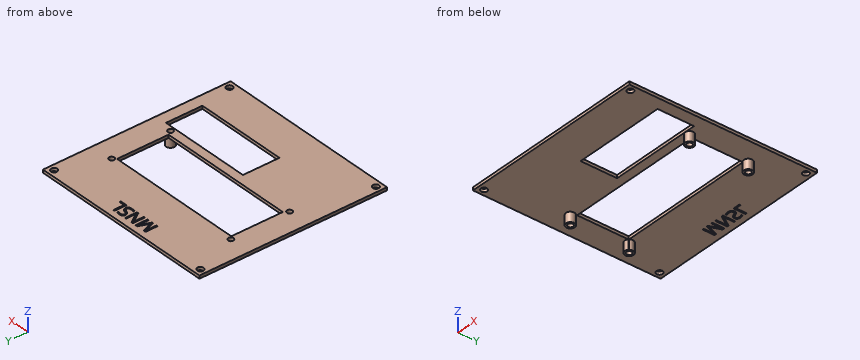
```python
from build123d import *

# Parameters (mm, degrees)
F0_W     = 98.044
F0_H     = 98.044
F0_R     = 1.651
F0_R_2   = 2.286
F0_R_3   = 1.397
F1_DEPTH = 1.5875
F2_DEPTH = 5.08


with BuildPart() as f1:
    # F0 (on Top) → F1 (new body)
    with BuildSketch(Plane.XY):
        Rectangle(F0_W, F0_H)
        with Locations((-45.847, -45.847)):
            Circle(F0_R, mode=Mode.SUBTRACT)
        with Locations((-37.338, -7.874)):
            Circle(F0_R_2, mode=Mode.SUBTRACT)
        with Locations((45.847, -45.847)):
            Circle(F0_R, mode=Mode.SUBTRACT)
        Polygon((-5.334, -29.21), (-5.334, -10.16), (37.3379999666, -10.16), (42.926, -10.16), (42.926, -29.21), align=None, mode=Mode.SUBTRACT)
        with BuildLine():
            ThreePointArc((39.624, -7.874), (38.95444609, -9.4904461136), (37.3379999666, -10.16))
            ThreePointArc((37.3379999666, -10.16), (35.72155391, -6.2575538864), (39.624, -7.874))
        make_face(mode=Mode.SUBTRACT)
        with Locations((-45.847, 45.847)):
            Circle(F0_R, mode=Mode.SUBTRACT)
        with BuildLine():
            Line((-7.9581705729, 39.497), (-8.5479709201, 39.497))
            Line((-8.5479709201, 39.497), (-10.6839301215, 45.0780546875))
            Line((-10.6839301215, 45.0780546875), (-10.7183810764, 45.0780546875))
            add(Edge.make_bspline(
                [(-10.7183810764, 45.0780546875), (-10.6577473958, 44.415218316), (-10.6577473958, 43.5015789931)],
                knots=[0, 0, 0, 1, 1, 1], degree=2))
            Line((-10.6577473958, 43.5015789931), (-10.6577473958, 39.497))
            Line((-10.6577473958, 39.497), (-11.3343641493, 39.497))
            Line((-11.3343641493, 39.497), (-11.3343641493, 45.7932565104))
            Line((-11.3343641493, 45.7932565104), (-10.2319335938, 45.7932565104))
            Line((-10.2319335938, 45.7932565104), (-8.2379123264, 40.5994305556))
            Line((-8.2379123264, 40.5994305556), (-8.2034613715, 40.5994305556))
            Line((-8.2034613715, 40.5994305556), (-6.1929036458, 45.7932565104))
            Line((-6.1929036458, 45.7932565104), (-5.0987413194, 45.7932565104))
            Line((-5.0987413194, 45.7932565104), (-5.0987413194, 39.497))
            Line((-5.0987413194, 39.497), (-5.8304796007, 39.497))
            Line((-5.8304796007, 39.497), (-5.8304796007, 43.5539444444))
            add(Edge.make_bspline(
                [(-5.8304796007, 43.5539444444), (-5.8304796007, 44.2512317708), (-5.7698459201, 45.0697864583)],
                knots=[0, 0, 0, 1, 1, 1], degree=2))
            Line((-5.7698459201, 45.0697864583), (-5.804296875, 45.0697864583))
            Line((-5.804296875, 45.0697864583), (-7.9581705729, 39.497))
        make_face(mode=Mode.SUBTRACT)
        with BuildLine():
            Line((1.5461588542, 45.7932565104), (1.5461588542, 39.497))
            Line((1.5461588542, 39.497), (0.7110677083, 39.497))
            Line((0.7110677083, 39.497), (-2.7298936632, 44.7803984375))
            Line((-2.7298936632, 44.7803984375), (-2.7643446181, 44.7803984375))
            add(Edge.make_bspline(
                [(-2.7643446181, 44.7803984375), (-2.6954427083, 43.8502226563), (-2.6954427083, 43.075765191)],
                knots=[0, 0, 0, 1, 1, 1], degree=2))
            Line((-2.6954427083, 43.075765191), (-2.6954427083, 39.497))
            Line((-2.6954427083, 39.497), (-3.3720594618, 39.497))
            Line((-3.3720594618, 39.497), (-3.3720594618, 45.7932565104))
            Line((-3.3720594618, 45.7932565104), (-2.5452365451, 45.7932565104))
            Line((-2.5452365451, 45.7932565104), (0.8874565972, 40.5305286458))
            Line((0.8874565972, 40.5305286458), (0.9219075521, 40.5305286458))
            add(Edge.make_bspline(
                [(0.9219075521, 40.5305286458), (0.9136393229, 40.6462838542), (0.8833224826, 41.2774253472)],
                knots=[0, 0, 0, 1, 1, 1], degree=2))
            add(Edge.make_bspline(
                [(0.8833224826, 41.2774253472), (0.8530056424, 41.9085668403), (0.8612738715, 42.1800403646)],
                knots=[0, 0, 0, 1, 1, 1], degree=2))
            Line((0.8612738715, 42.1800403646), (0.8612738715, 45.7932565104))
            Line((0.8612738715, 45.7932565104), (1.5461588542, 45.7932565104))
        make_face(mode=Mode.SUBTRACT)
        with BuildLine():
            ThreePointArc((-35.814, 21.1561162011), (-39.4248229441, 23.793255592), (-35.052, 22.86))
            ThreePointArc((-35.052, 22.86), (-35.2024819874, 22.0443047028), (-35.6341162011, 21.336))
            Line((-35.6341162011, 21.336), (35.6341162011, 21.336))
            ThreePointArc((35.6341162011, 21.336), (36.5223047028, 24.9955180126), (39.624, 22.86))
            ThreePointArc((39.624, 22.86), (38.271255592, 20.7731770559), (35.814, 21.1561162011))
            Line((35.814, 21.1561162011), (35.814, -5.588))
            Line((35.814, -5.588), (-35.814, -5.588))
            Line((-35.814, -5.588), (-35.814, 21.1561162011))
        make_face(mode=Mode.SUBTRACT)
        with BuildLine():
            add(Edge.make_bspline(
                [(6.4574869792, 42.2227595486), (6.8295572917, 41.8176163194), (6.8295572917, 41.1726944444)],
                knots=[0, 0, 0, 1, 1, 1], degree=2))
            add(Edge.make_bspline(
                [(6.8295572917, 41.1726944444), (6.8295572917, 40.3417374132), (6.2266655816, 39.8759605035)],
                knots=[0, 0, 0, 1, 1, 1], degree=2))
            add(Edge.make_bspline(
                [(6.2266655816, 39.8759605035), (5.6237738715, 39.4101835938), (4.5902452257, 39.4101835938)],
                knots=[0, 0, 0, 1, 1, 1], degree=2))
            add(Edge.make_bspline(
                [(4.5902452257, 39.4101835938), (3.4712782118, 39.4101835938), (2.8676974826, 39.6995716146)],
                knots=[0, 0, 0, 1, 1, 1], degree=2))
            Line((2.8676974826, 39.6995716146), (2.8676974826, 40.4051271701))
            add(Edge.make_bspline(
                [(2.8676974826, 40.4051271701), (3.2563042535, 40.2425186632), (3.7124348958, 40.1474340278)],
                knots=[0, 0, 0, 1, 1, 1], degree=2))
            add(Edge.make_bspline(
                [(3.7124348958, 40.1474340278), (4.1685655382, 40.0523493924), (4.6164279514, 40.0523493924)],
                knots=[0, 0, 0, 1, 1, 1], degree=2))
            add(Edge.make_bspline(
                [(4.6164279514, 40.0523493924), (5.3481662326, 40.0523493924), (5.7188585069, 40.3300240885)],
                knots=[0, 0, 0, 1, 1, 1], degree=2))
            add(Edge.make_bspline(
                [(5.7188585069, 40.3300240885), (6.0895507813, 40.6076987847), (6.0895507813, 41.1037925347)],
                knots=[0, 0, 0, 1, 1, 1], degree=2))
            add(Edge.make_bspline(
                [(6.0895507813, 41.1037925347), (6.0895507813, 41.4303875868), (5.9579481337, 41.6391603733)],
                knots=[0, 0, 0, 1, 1, 1], degree=2))
            add(Edge.make_bspline(
                [(5.9579481337, 41.6391603733), (5.8263454861, 41.8479331597), (5.5183539497, 42.0250110677)],
                knots=[0, 0, 0, 1, 1, 1], degree=2))
            add(Edge.make_bspline(
                [(5.5183539497, 42.0250110677), (5.2103624132, 42.2020889757), (4.5819769965, 42.4253311632)],
                knots=[0, 0, 0, 1, 1, 1], degree=2))
            add(Edge.make_bspline(
                [(4.5819769965, 42.4253311632), (3.7041666667, 42.7395238715), (3.3272732205, 43.1701608073)],
                knots=[0, 0, 0, 1, 1, 1], degree=2))
            add(Edge.make_bspline(
                [(3.3272732205, 43.1701608073), (2.9503797743, 43.6007977431), (2.9503797743, 44.2939509549)],
                knots=[0, 0, 0, 1, 1, 1], degree=2))
            add(Edge.make_bspline(
                [(2.9503797743, 44.2939509549), (2.9503797743, 45.0215551215), (3.4967719184, 45.4521920573)],
                knots=[0, 0, 0, 1, 1, 1], degree=2))
            add(Edge.make_bspline(
                [(3.4967719184, 45.4521920573), (4.0431640625, 45.8828289931), (4.9444010417, 45.8828289931)],
                knots=[0, 0, 0, 1, 1, 1], degree=2))
            add(Edge.make_bspline(
                [(4.9444010417, 45.8828289931), (5.8828450521, 45.8828289931), (6.6710828993, 45.5383194444)],
                knots=[0, 0, 0, 1, 1, 1], degree=2))
            Line((6.6710828993, 45.5383194444), (6.442328559, 44.9016657986))
            add(Edge.make_bspline(
                [(6.442328559, 44.9016657986), (5.662358941, 45.2282608507), (4.9264865451, 45.2282608507)],
                knots=[0, 0, 0, 1, 1, 1], degree=2))
            add(Edge.make_bspline(
                [(4.9264865451, 45.2282608507), (4.3449544271, 45.2282608507), (4.0176703559, 44.9788359375)],
                knots=[0, 0, 0, 1, 1, 1], degree=2))
            add(Edge.make_bspline(
                [(4.0176703559, 44.9788359375), (3.6903862847, 44.7294110243), (3.6903862847, 44.2856827257)],
                knots=[0, 0, 0, 1, 1, 1], degree=2))
            add(Edge.make_bspline(
                [(3.6903862847, 44.2856827257), (3.6903862847, 43.9590876736), (3.8109646267, 43.7496258681)],
                knots=[0, 0, 0, 1, 1, 1], degree=2))
            add(Edge.make_bspline(
                [(3.8109646267, 43.7496258681), (3.9315429688, 43.5401640625), (4.2181749132, 43.3658422309)],
                knots=[0, 0, 0, 1, 1, 1], degree=2))
            add(Edge.make_bspline(
                [(4.2181749132, 43.3658422309), (4.5048068576, 43.1915203993), (5.0946072049, 42.9806805556)],
                knots=[0, 0, 0, 1, 1, 1], degree=2))
            add(Edge.make_bspline(
                [(5.0946072049, 42.9806805556), (6.0854166667, 42.6279027778), (6.4574869792, 42.2227595486)],
                knots=[0, 0, 0, 1, 1, 1], degree=2))
        make_face(mode=Mode.SUBTRACT)
        Polygon((11.6278862847, 39.497), (8.1180230035, 39.497), (8.1180230035, 45.7932565104), (8.8497612847, 45.7932565104), (8.8497612847, 40.1598363715), (11.6278862847, 40.1598363715), align=None, mode=Mode.SUBTRACT)
        with Locations((45.847, 45.847)):
            Circle(F0_R, mode=Mode.SUBTRACT)
        with Locations((-37.338, -7.874)):
            Circle(F0_R_2)
        with Locations((-37.338, -7.874)):
            Circle(F0_R_3, mode=Mode.SUBTRACT)
        with BuildLine():
            ThreePointArc((39.624, -7.874), (35.72155391, -6.2575538864), (37.3379999666, -10.16))
            ThreePointArc((37.3379999666, -10.16), (38.95444609, -9.4904461136), (39.624, -7.874))
        make_face()
        with Locations((37.338, -7.874)):
            Circle(F0_R_3, mode=Mode.SUBTRACT)
        with BuildLine():
            ThreePointArc((39.624, 22.86), (36.5223047028, 24.9955180126), (35.6341162011, 21.336))
            Line((35.6341162011, 21.336), (35.814, 21.336))
            Line((35.814, 21.336), (35.814, 21.1561162011))
            ThreePointArc((35.814, 21.1561162011), (38.271255592, 20.7731770559), (39.624, 22.86))
        make_face()
        with Locations((37.338, 22.86)):
            Circle(F0_R_3, mode=Mode.SUBTRACT)
        with BuildLine():
            ThreePointArc((-35.6341162011, 21.336), (-35.2024819874, 22.0443047028), (-35.052, 22.86))
            ThreePointArc((-35.052, 22.86), (-39.4248229441, 23.793255592), (-35.814, 21.1561162011))
            Line((-35.814, 21.1561162011), (-35.814, 21.336))
            Line((-35.814, 21.336), (-35.6341162011, 21.336))
        make_face()
        with Locations((-37.338, 22.86)):
            Circle(F0_R_3, mode=Mode.SUBTRACT)
    extrude(amount=F1_DEPTH)

    # F0 (on Top) → F2 (join)
    with BuildSketch(Plane.XY):
        with BuildLine():
            ThreePointArc((39.624, 22.86), (36.5223047028, 24.9955180126), (35.6341162011, 21.336))
            Line((35.6341162011, 21.336), (35.814, 21.336))
            Line((35.814, 21.336), (35.814, 21.1561162011))
            ThreePointArc((35.814, 21.1561162011), (38.271255592, 20.7731770559), (39.624, 22.86))
        make_face()
        with Locations((37.338, 22.86)):
            Circle(F0_R_3, mode=Mode.SUBTRACT)
        with Locations((-37.338, -7.874)):
            Circle(F0_R_2)
        with Locations((-37.338, -7.874)):
            Circle(F0_R_3, mode=Mode.SUBTRACT)
        with BuildLine():
            ThreePointArc((-35.6341162011, 21.336), (-35.2024819874, 22.0443047028), (-35.052, 22.86))
            ThreePointArc((-35.052, 22.86), (-39.4248229441, 23.793255592), (-35.814, 21.1561162011))
            Line((-35.814, 21.1561162011), (-35.814, 21.336))
            Line((-35.814, 21.336), (-35.6341162011, 21.336))
        make_face()
        with Locations((-37.338, 22.86)):
            Circle(F0_R_3, mode=Mode.SUBTRACT)
        with BuildLine():
            ThreePointArc((39.624, -7.874), (35.72155391, -6.2575538864), (37.3379999666, -10.16))
            ThreePointArc((37.3379999666, -10.16), (38.95444609, -9.4904461136), (39.624, -7.874))
        make_face()
        with Locations((37.338, -7.874)):
            Circle(F0_R_3, mode=Mode.SUBTRACT)
    extrude(amount=-F2_DEPTH)


solid = f1.part
```
The listing builds one solid part. Answer for the finished solid, in the listing's coordinates (mm). Give positions to 0.01 mm unless a question says otherwise; leave off trailing zeros. Loops run counter-clockwise (first coordinate to the right, second up) from the corner with the lowest first, then second, coordinate; pieces in that order, holes last. Notation, with made-up numbers: (5.25, 2) - (16.25, 2) arc R16 ccw to (16.25, 16) - close; hole circle Ø1 at (74.25, 51). An arc over 180 degrees is marked (long way). Answer as CSV lines item,"result". Start each with the question number.
Item 1: A cutting plane is placed at D-D on z = -2. Determine the outline of the cut face in (x, y) (3 decimals).
Item 2: A cutting plane is placed at A-A on y = -4. Determine the outline of the cut face in (x, z), then the cut area to 3 significant figures.
Item 3: A cutting plane is placed at C-C on x = 31.5. Determine the outline of the cut face in (y, z), then the cut area to 3 significant figures.
Item 4: A cutting plane is placed at B-B on x = -19.5. Determine the outline of the cut face in (y, z).
Item 5: Find the intervals of material crossed by line 1 (Y direction, x = 21.5, z = 0.75); line 2 (X direction, y = 24, z = -2); line 3 (X direction, y = 5, z = 1.25), in increasing order. Write a range as from..to.
Item 6: This flat-tipped pin is pushed along its axis until it touches: pin 1 (2 mm diameter, centred on x = 34.5, y = -30, fed in from -Z). Where does it stop, or does it pass through?
Found:
1,outline,"circle Ø4.572 at (-37.338, -7.874); (-35.814, 21.156) - (-35.814, 21.336) - (-35.634, 21.336) arc R2.286 ccw (long way) to start; circle Ø4.572 at (37.338, -7.874); (35.634, 21.336) - (35.814, 21.336) - (35.814, 21.156) arc R2.286 ccw (long way) to start; hole circle Ø2.794 at (-37.338, -7.874); hole circle Ø2.794 at (-37.338, 22.86); hole circle Ø2.794 at (37.338, -7.874); hole circle Ø2.794 at (37.338, 22.86)"
2,outline,"(-49.02, 0) - (-35.81, 0) - (-35.81, 1.59) - (-49.02, 1.59) - close; (35.81, 0) - (49.02, 0) - (49.02, 1.59) - (35.81, 1.59) - close"
2,area,"41.9 mm^2"
3,outline,"(-49.02, 0) - (-29.21, 0) - (-29.21, 1.59) - (-49.02, 1.59) - close; (-10.16, 0) - (-5.59, 0) - (-5.59, 1.59) - (-10.16, 1.59) - close; (21.34, 0) - (49.02, 0) - (49.02, 1.59) - (21.34, 1.59) - close"
3,area,"82.7 mm^2"
4,outline,"(-49.02, 0) - (-5.59, 0) - (-5.59, 1.59) - (-49.02, 1.59) - close; (21.34, 0) - (49.02, 0) - (49.02, 1.59) - (21.34, 1.59) - close"
5,line 1,"y = -49.02..-29.21, -10.16..-5.59, 21.34..49.02"
5,line 2,"x = -39.32..-38.15, -36.53..-35.36, 35.36..36.53, 38.15..39.32"
5,line 3,"x = -49.02..-35.81, 35.81..49.02"
6,pin 1,"stops at z = 0"
